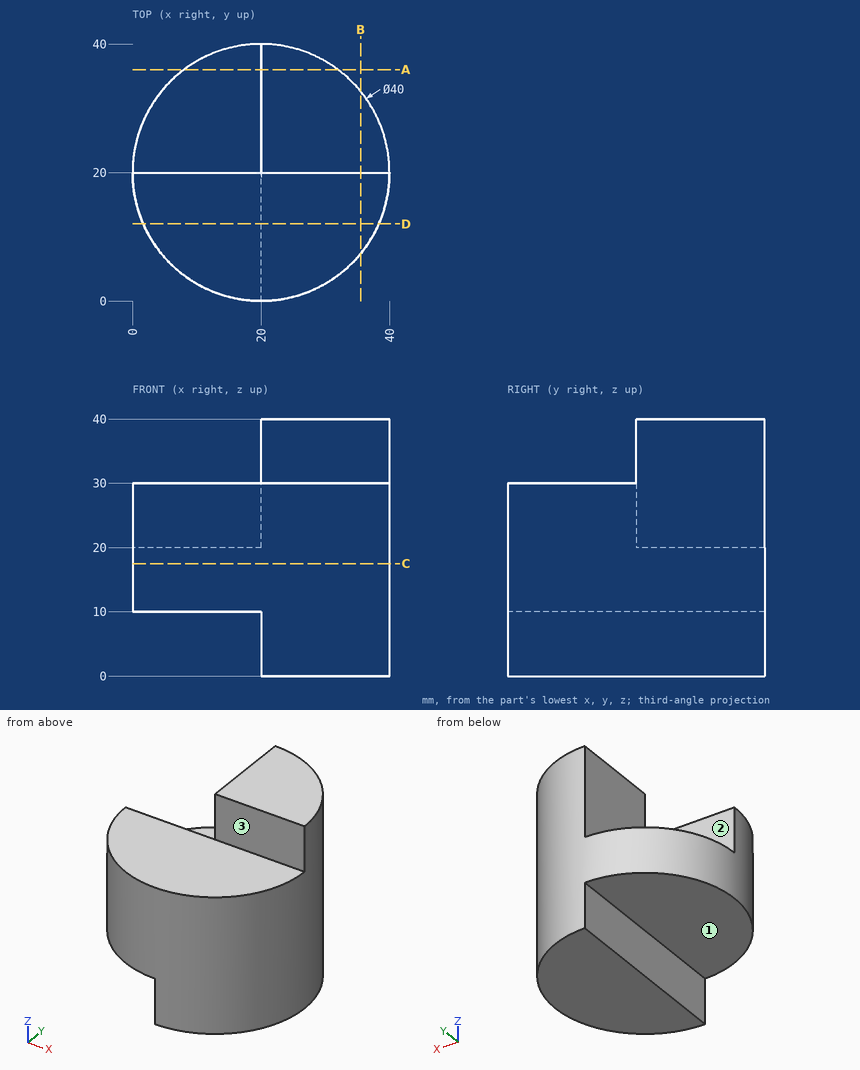
Input: dimensioned drawing with shaded views. Units: mm. Origin: part minimum x, y, z. A direction names the side the tool comes from. Coordinates: 2 decimals unless noted, no trailing zeros. Order: outer loops, then holes, each group sorted by start corner. A loop starts at its lowest first (then second) coordinate and runs counter-clockwise, first axis right, second up.
Item 1: Section query A-A (y = 36). Output: boundary loops of the cut face in (x, z), then the cut area to 3 significant figures.
Answer:
outline: (8, 10) - (20, 10) - (20, 0) - (32, 0) - (32, 40) - (20, 40) - (20, 20) - (8, 20) - close
area: 600 mm2
Item 2: Access query for the marked faces 1, 2 and 3. Directions: +Z, -Z, +X, -X, +Y, -Y. A direction counts if a zero-diameter tool reaches every point of the face in a straight line with its end or side. Return the directions, or none.
Answer:
face 1: -Z, -X, +Y, -Y
face 2: +Z, -X, +Y
face 3: +Z, +X, -X, -Y
Item 3: Material intervals for line 1 along Z through (x, y) = (9, 12.5); line 2 along Z through (x, y) = (11.5, 37); line 3 along X through (y, z) = (5.5, 18), sorted ascending.
Answer:
line 1: z = 10 to 30
line 2: z = 10 to 20
line 3: x = 6.23 to 33.77
Item 4: Section query B-B (x = 35.5). Output: boundary loops of the cut face in (y, z), then the cut area to 3 significant figures.
Answer:
outline: (7.36, 0) - (32.64, 0) - (32.64, 40) - (20, 40) - (20, 30) - (7.36, 30) - close
area: 885 mm2
Item 5: Contact query for flat-ended pins moving along their axis: P1, Ø3, axis at x = 30.5, y = 13, coming from the +Z side; P2, Ø8, axis at y = 24.5, z = 4, coming from the -X side; P3, Ø10, axis at x = 30, z = 7, coming from the -Y side. Output: stop coordinate, or through.
Answer:
P1: stops at z = 30
P2: stops at x = 20
P3: stops at y = 0.64
Item 6: Section query D-D (y = 12). Output: boundary loops of the cut face in (x, z), then the cut area to 3 significant figures.
Answer:
outline: (1.67, 10) - (20, 10) - (20, 0) - (38.33, 0) - (38.33, 30) - (1.67, 30) - close
area: 917 mm2
Item 7: Section query C-C (z = 17.5). Output: boundary loops of the cut face in (x, y), then the cut area to 3 significant figures.
Answer:
outline: circle Ø40 at (20, 20)
area: 1,260 mm2
